Autodesk Inventor part; units mm, degrees
ref_plane "YZ Plane" through (0, 0, 0) normal (1, 0, 0) x (0, 1, 0)
ref_plane "XZ Plane" through (0, 0, 0) normal (0, 1, 0) x (-1, 0, 0)
ref_plane "XY Plane" through (0, 0, 0) normal (0, 0, 1) x (1, 0, 0)
sketch "Sketch1" plane through (0, 0, 0) normal (0, 0, 1) x (1, 0, 0)
  line L0 (-12.1708, 16.0073) -> (13.2292, 16.0073)
  line L1 (13.2292, 16.0073) -> (13.2292, -34.7927)
  line L2 (13.2292, -34.7927) -> (-12.1708, -34.7927)
  line L3 (-12.1708, -34.7927) -> (-12.1708, 16.0073)
  line L4 (11.9592, 14.7373) -> (-10.9008, 14.7373)
  line L5 (-10.9008, 14.7373) -> (-10.9008, -33.5227)
  line L6 (-10.9008, -33.5227) -> (11.9592, -33.5227)
  line L7 (11.9592, -33.5227) -> (11.9592, 14.7373)
  point P0 (0, 0)
  dimension "d0" = 25.4
  dimension "d1" = 50.8
  dimension "d2" = 1.27
extrude "Extrusion1" add sketch "Sketch1" along normal blind 609.6
sketch "Sketch2" plane through (-12.1708, 16.0073, 0) normal (0, 1, 0) x (1, 0, 0)
  circle A0 centre (12.7, -12.7) radius 1.7272
  line L0 (25.4, 0) -> (0, 0)
  line L1 (0, 0) -> (0, -609.6)
  point P0 (12.1708, 0)
  dimension "d5" = 3.4544
  dimension "d6" = 12.7
  dimension "d7" = 12.7
extrude "Extrusion2" cut sketch "Sketch2" against normal through all
pattern_linear "Rectangular Pattern1" count 61 spacing 25.4 along (0, 0, 1) of "Extrusion2"
sketch "Sketch4" plane through (13.2292, -34.7927, 0) normal (1, 0, 0) x (0, 0, -1)
  circle A0 centre (-558.8, 25.4) radius 14.2875
  circle A1 centre (-50.8, 25.4) radius 14.2875
  line L0 (-609.6, 0) -> (-609.6, 50.8)
  line L1 (0, 0) -> (0, 50.8)
  point P0 (0, 34.7927)
  dimension "d19" = 28.575
  dimension "d20" = 28.575
  dimension "d21" = 50.8
  dimension "d22" = 50.8
extrude "Extrusion4" cut sketch "Sketch4" against normal through all
equation "\"d3\" = d13"
equation "\"d10\" = d14"
equation "\"d13\" = 609.6"
equation "\"d14\" = d13"
properties part number "Elevator Versaframe2"
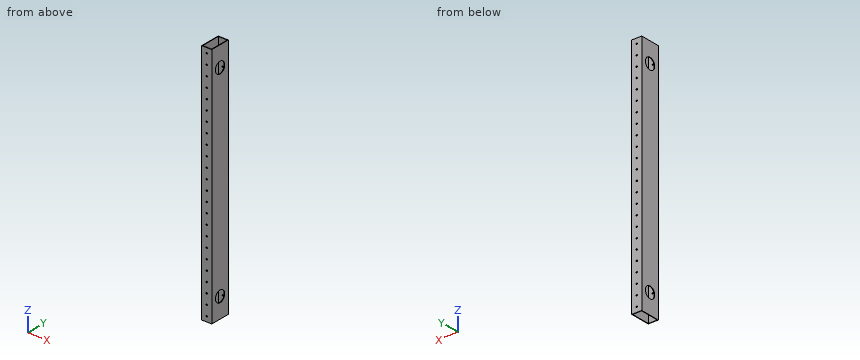
Geometry check sheet. Reference: the model listing, model coordinates, mm. Give positions to 0.01 mm unless a question says otherwise; leave off trailing zeros. Loops run counter-clockwise (first coordinate to the right, second up) from the corner with the lowest first, then second, coordinate; pieces in that order, holes last. Notation, with made-up numbers: M 54.5,43 L 88.5,43 A33 cw 88.5,80 Z; hole C 42,76 d7. An arc over 180 degrees is marked long. Write item = value, one per line. Start each with the question number.
1. Section check C-C, the plane z = 483. Enter the section's corners in (x, y), plus the area to 3 significant figures.
2. Thickness scan on probe 1 along Y at (x, z) = (9.75, 518.5); probe 2 along X at (y, z) = (-23.5, 280.5); probe 3 along X at (y, z) = (15.5, 317.5). Record the ranges inside material, lowest first.
3. Section check B-B, the plane z = 558.8. Enter the section's corners in (x, y), plus the area to 3 significant figures.
4. Section check A-A, the plane x = -6.75. Enter the section's corners in (y, z).
Values follow:
q1.outline = M -12.17,-34.79 L 13.23,-34.79 L 13.23,16.01 L -12.17,16.01 Z; hole M -10.9,-33.52 L 11.96,-33.52 L 11.96,14.74 L -10.9,14.74 Z
q1.area = 187 mm^2
q2.probe_1 = -34.79 to -33.52, 14.74 to 16.01
q2.probe_2 = -12.17 to -10.9, 11.96 to 13.23
q2.probe_3 = -12.17 to -1.2, 2.26 to 13.23
q3.outline = M -12.17,-34.79 L 13.23,-34.79 L 13.23,-23.68 L 11.96,-23.68 L 11.96,-33.52 L -10.9,-33.52 L -10.9,-23.68 L -12.17,-23.68 Z; M -12.17,4.89 L -10.9,4.89 L -10.9,14.74 L 11.96,14.74 L 11.96,4.89 L 13.23,4.89 L 13.23,16.01 L -12.17,16.01 Z
q3.area = 115 mm^2
q4.outline = M -34.79,0 L -33.52,0 L -33.52,609.6 L -34.79,609.6 Z; M 14.74,0 L 16.01,0 L 16.01,609.6 L 14.74,609.6 Z
